Autodesk Inventor part; units mm, degrees
ref_plane "Work Plane1" through (-215.9, 0, 285.75) normal (1, 0, 0) x (0, 0, -1)
ref_plane "YZ Plane" through (0, 0, 0) normal (1, 0, 0) x (0, 1, 0)
ref_plane "XZ Plane" through (0, 0, 0) normal (0, 1, 0) x (-1, 0, 0)
sketch "Sketch1" plane through (0, 0, 0) normal (0, 1, 0) x (-1, 0, 0)
  line L0 (0, 0) -> (431.8, 0)
  line L1 (431.8, 0) -> (431.8, 361.95)
  line L2 (431.8, 361.95) -> (0, 361.95)
  line L3 (0, 361.95) -> (0, 0)
  dimension "d0" = 431.8
  dimension "d1" = 361.95
extrude "Extrusion1" add sketch "Sketch1" along normal blind 6.35
sketch "Sketch3" plane through (0, 6.35, 0) normal (0, 1, 0) x (1, 0, 0)
  line L0 (-431.8, 0) -> (-431.8, -361.95)
  line L1 (-431.8, -361.95) -> (-381, -361.95)
  line L2 (-381, -361.95) -> (-381, -285.75)
  line L3 (-381, -285.75) -> (-431.8, -285.75)
  line L4 (-431.8, -285.75) -> (-431.8, -361.95)
  line L5 (-431.8, -38.1) -> (-381, -38.1)
  line L6 (-381, -38.1) -> (-381, -127)
  line L7 (-381, -127) -> (-431.8, -127)
  line L8 (-431.8, -127) -> (-431.8, -38.1)
  line L9 (0, -361.95) -> (0, 0)
  line L10 (0, -38.1) -> (-50.8, -38.1)
  line L11 (-50.8, -38.1) -> (-50.8, -127)
  line L12 (-50.8, -127) -> (0, -127)
  line L13 (0, -127) -> (0, -38.1)
  line L14 (0, -361.95) -> (-50.8, -361.95)
  line L15 (-50.8, -361.95) -> (-50.8, -285.75)
  line L16 (-50.8, -285.75) -> (0, -285.75)
  line L17 (0, -285.75) -> (0, -361.95)
  line L18 (0, 0) -> (-431.8, 0)
  dimension "d11" = 76.2
  dimension "d12" = 88.9
  dimension "d13" = 127
  dimension "d14" = 50.8
  dimension "d15" = 50.8
extrude "Extrusion3" cut sketch "Sketch3" against normal blind 6.35
sketch "Sketch4" plane through (0, 6.35, 0) normal (0, 1, 0) x (1, 0, 0)
  line L0 (0, 0) -> (-431.8, 0)
  line L1 (-381, -38.1) -> (-381, -127)
  line L2 (-381, -285.75) -> (-381, -361.95)
  line L3 (-381, -361.95) -> (-50.8, -361.95)
  point P0 (-375.0056, -66.294)
  point P1 (-375.0056, -98.298)
  point P2 (-314.0964, -66.294)
  point P3 (-314.0964, -98.298)
  point P4 (-375.0056, -345.948)
  point P5 (-375.0056, -313.944)
  point P6 (-314.0964, -345.948)
  point P7 (-314.0964, -313.944)
  dimension "d18" = 66.294
  dimension "d19" = 5.9944
  dimension "d20" = 98.298
  dimension "d21" = 5.9944
  dimension "d22" = 66.9036
  dimension "d23" = 66.294
  dimension "d24" = 98.298
  dimension "d25" = 66.9036
  dimension "d26" = 5.9944
  dimension "d27" = 16.002
  dimension "d28" = 5.9944
  dimension "d29" = 48.006
  dimension "d30" = 66.9036
  dimension "d31" = 66.9036
  dimension "d32" = 16.002
  dimension "d33" = 48.006
hole "Hole1" at (-375.0056, 6.35, 66.294) at (-375.0056, 6.35, 98.298) at (-314.0964, 6.35, 66.294) at (-314.0964, 6.35, 98.298) at (-375.0056, 6.35, 345.948) at (-375.0056, 6.35, 313.944) at (-314.0964, 6.35, 345.948) at (-314.0964, 6.35, 313.944) direction (0, -1, 0) diameter 3.81 end through all
ref_plane "Work Plane1" through (-215.9, 0, 285.75) normal (1, 0, 0) x (0, 0, -1)
mirror "Mirror1" about plane through (-215.9, 0, 285.75) normal (1, 0, 0) of "Hole1"
properties part number "Gen 2.0 rev mecanums base plate"
Read the model definition and answer for the solid it produces. Units are mm, in the model's axes. Round coordinates to 2 decimals unless told otherwise and drop trailing zeros. Write each loop counter-clockwise with the first axis right and the second up, starting at its lowest first coordinate (ties: lowest second). Pieces come first, ordered by that corner, then holes. Notation, with made-up numbers: (14.5, 30.25) -> (66.5, 30.25) arc R22 ccw to (66.5, 38.25) -> close; hole circle Ø3 at (14, -31.75). An arc over 180 degrees is marked (long way). Answer in a Markdown table with one row per item. Add a question column.
1) Find section B-B, the plane y = 1. State how many separate pieces and enclosed holes the cut face has, and give its area (3 significant figures).
2) Find section C-C, the plane z = 297. Determine the outline of the cut face in (x, y), and give its area (3 significant figures).
3) Find section A-A, the plane x = -45. Determine the outline of the cut face in (y, z).
4) Consider line 1 (Z direction, x = -396, y = 5.75); line 2 (X direction, y = 4.75, z = 89.5). Determine where each line is inside the solid, lowest interval first.
Findings below:
| question | item | result |
|---|---|---|
| 1 | separate pieces | 1 |
| 1 | enclosed holes | 16 |
| 1 | area | 139,000 mm² |
| 2 | outline | (-381, 0) -> (-50.8, 0) -> (-50.8, 6.35) -> (-381, 6.35) -> close |
| 2 | area | 2,100 mm² |
| 3 | outline | (0, 0) -> (6.35, 0) -> (6.35, 38.1) -> (0, 38.1) -> close; (0, 127) -> (6.35, 127) -> (6.35, 285.75) -> (0, 285.75) -> close |
| 4 | line 1 | 0 to 38.1, 127 to 285.75 |
| 4 | line 2 | -381 to -50.8 |
